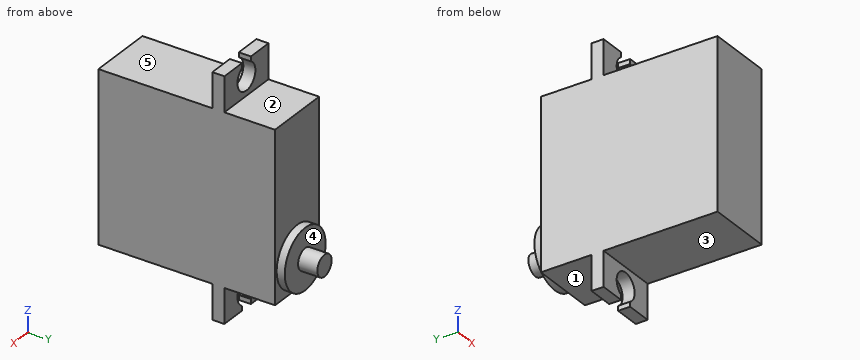
from build123d import *

# Parameters (mm, degrees)
SKETCH1_W           = 10.8
SKETCH1_H           = 28
BOSS_EXTRUDE1_DEPTH = 29.3
BOSS_EXTRUDE2_DEPTH = 2
SKETCH3_R           = 5
BOSS_EXTRUDE3_DEPTH = 1.35
SKETCH4_R           = 1.75
BOSS_EXTRUDE4_DEPTH = 3.2


with BuildPart() as part:
    # Sketch1 → Boss-Extrude1 (new body)
    with BuildSketch(Plane(origin=(0, 0, 0), x_dir=(1, 0, 0), z_dir=(0, 1, 0))):
        with Locations((5.4, 14)):
            Rectangle(SKETCH1_W, SKETCH1_H)
    extrude(amount=BOSS_EXTRUDE1_DEPTH)

    # Sketch2 → Boss-Extrude2 (add)
    with BuildSketch(Plane(origin=(0, 20.9, 0), x_dir=(1, 0, 0), z_dir=(0, 1, 0))):
        with BuildLine():
            Line((0, 28), (10.8, 28))
            Line((10.8, 28), (10.8, 33.75))
            Line((10.8, 33.75), (6.5, 33.75))
            Line((6.5, 33.75), (6.5, 32.955255888))
            ThreePointArc((6.5, 32.955255888), (5.4, 28.85), (4.3, 32.955255888))
            Line((4.3, 32.955255888), (4.3, 33.75))
            Line((4.3, 33.75), (0, 33.75))
            Line((0, 33.75), (0, 28))
        make_face()
        with BuildLine():
            Line((10.8, 0), (10.8, -5.75))
            Line((10.8, -5.75), (6.5, -5.75))
            Line((6.5, -5.75), (6.5, -4.955255888))
            ThreePointArc((6.5, -4.955255888), (5.4, -0.85), (4.3, -4.955255888))
            Line((4.3, -4.955255888), (4.3, -5.75))
            Line((4.3, -5.75), (0, -5.75))
            Line((0, -5.75), (0, 0))
            Line((0, 0), (10.8, 0))
        make_face()
    extrude(amount=-BOSS_EXTRUDE2_DEPTH)

    # Sketch3 → Boss-Extrude3 (add)
    with BuildSketch(Plane(origin=(0, 29.3, 0), x_dir=(1, 0, 0), z_dir=(0, 1, 0))):
        with Locations(Location((5.4, 22.8, 0), (0, 0, 90))):
            Circle(SKETCH3_R)
    extrude(amount=BOSS_EXTRUDE3_DEPTH)

    # Sketch4 → Boss-Extrude4 (add)
    with BuildSketch(Plane(origin=(0, 30.65, 0), x_dir=(1, 0, 0), z_dir=(0, 1, 0))):
        with Locations(Location((5.4, 22.8, 0), (0, 0, 270))):
            Circle(SKETCH4_R)
    extrude(amount=BOSS_EXTRUDE4_DEPTH)


solid = part.part
Here's how the part is built. I have some questions about the finished solid (model axes, mm). Face numbers are marked on the shaded views. A direction names the side the tool comes from. Give positions to 0.01 mm unless a question says otherwise; leave off trailing zeros. Order: outer loops, then holes, each group sorted by start corner. A loop starts at its lowest first (then second) coordinate and runs counter-clockwise, first axis right, second up. Notation, with made-up numbers: (2, -3) -> (28, -3) arc R34 ccw to (28, 30) -> close; hole circle Ø10 at (44.5, -26.5). An arc over 180 degrees is marked (long way). One line per item, written item: value. Start each with the question number.
1. Will these pins go through, and if not, where does the flat tip stop? pin 1 Ø6 at (y, z) = (30, -15.5) entering from +X; pin 2 Ø2 at (x, z) = (7, 1.5) entering from +Y; pin 3 Ø1.5 at (x, z) = (1.5, -7) entering from +Y; pin 4 Ø3.5 at (x, z) = (5.4, -31.05) entering from -Y.
2. For the marked faces 1, 2, 3, 4 and 5, which set-ups out of +Z, -Z, +X, -X, +Y, -Y let a thin tool reach every point of the face, with its end or its side?
3. Imagine slicing it at C-C, the plane z = -22.8. List the corners of the cut face in (x, y) for me, plus the area to 3 significant figures.
4. Imagine slicing it at D-D, the plane y = 11. List the corners of the cut face in (x, z) for me.
5. Imagine slicing it at A-A, the plane z = -31.05. List the corners of the cut face in (x, y) for me, plus the area to 3 significant figures.
6. Imagine slicing it at B-B, the plane x = 5.4. List the corners of the cut face in (y, z) for me.
7. I need wall thicknesses on probe 1 along X at (y, z) = (19.8, 3.05); probe 2 along Z at (x, y) = (3.75, 8); probe 3 along Z at (x, y) = (5.4, 20.1). Which ranges of each line are inside material? Lowest first, please. Write a range as from..to.
Values follow:
1. pin 1: stops at x = 10.8
1. pin 2: stops at y = 20.9
1. pin 3: stops at y = 29.3
1. pin 4: passes through
2. face 1: -Z, +X, -X, +Y
2. face 2: +Z, +X, -X, +Y
2. face 3: -Z, +X, -X, -Y
2. face 4: +Y
2. face 5: +Z, +X, -X, -Y
3. outline: (0, 0) -> (10.8, 0) -> (10.8, 29.3) -> (10.4, 29.3) -> (10.4, 30.65) -> (7.15, 30.65) -> (7.15, 33.85) -> (3.65, 33.85) -> (3.65, 30.65) -> (0.4, 30.65) -> (0.4, 29.3) -> (0, 29.3) -> close
3. area: 341 mm2
4. outline: (0, -28) -> (10.8, -28) -> (10.8, 0) -> (0, 0) -> close
5. outline: (0, 18.9) -> (3.2, 18.9) -> (3.2, 20.9) -> (0, 20.9) -> close; (7.6, 18.9) -> (10.8, 18.9) -> (10.8, 20.9) -> (7.6, 20.9) -> close
5. area: 12.8 mm2
6. outline: (0, -28) -> (18.9, -28) -> (18.9, -28.85) -> (20.9, -28.85) -> (20.9, -28) -> (29.3, -28) -> (29.3, -27.8) -> (30.65, -27.8) -> (30.65, -24.55) -> (33.85, -24.55) -> (33.85, -21.05) -> (30.65, -21.05) -> (30.65, -17.8) -> (29.3, -17.8) -> (29.3, 0) -> (20.9, 0) -> (20.9, 0.85) -> (18.9, 0.85) -> (18.9, 0) -> (0, 0) -> close
7. probe 1: x = 0..3.2, 7.6..10.8
7. probe 2: z = -28..0
7. probe 3: z = -28.85..0.85
